For this review, use the dimensioned drawing (mm, ordinates from the lowest corner) and the shaded views. A direction names the side the tool comes from. Round coordinates to 2 decimals unless told otherwise and drop trailing zeros. Loops run counter-clockwise (first coordinate to the right, second up) from the corner with the lowest first, then second, coordinate; pieces in that order, holes last.
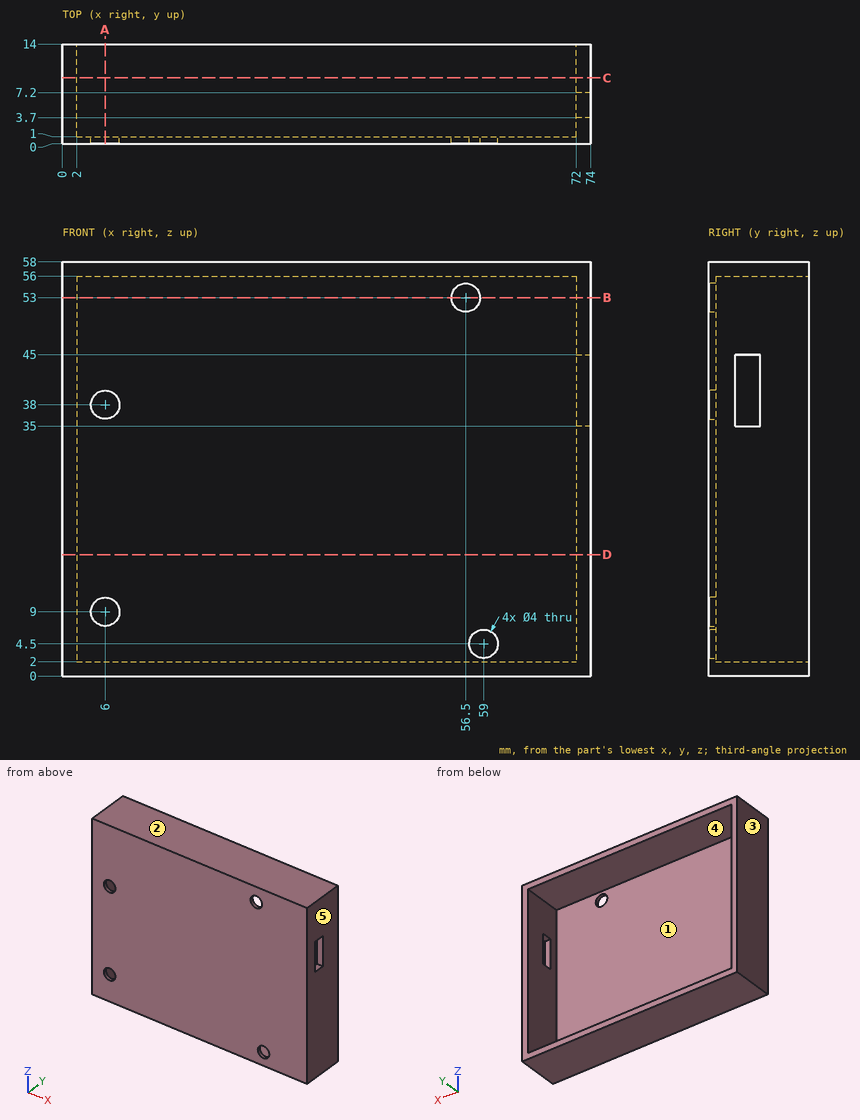
(1) Add section A-A (x = 6). Give the boundary of the cut face in (y, z).
(2) The part is to be moulded in two halves that separate along X. For the marked faces 3, 4 and 5, say which applies: pulls with the +X half, pulls with the -X half, needs draft (parallel to the pull), parting line crosses it, or undercut.
(3) For L1, parallel to X at y = 0.7, z = 9; L2, parallel to X at y = 12.75, z = 52; L3, parallel to Z at x = 56.5, y = 2, list the stretches that pass through material, from the lowest coordinate up.
(4) Add section D-D (z = 17). Give the boundary of the cut face in (x, y), plus the area to 3 significant figures.
(5) Insertion check: pin 1 Ø5 at (x, z) = (6, 9) entering from +Y; pin 2 Ø2.5 at (x, z) = (56.5, 53) entering from +Y. Each pin has a flat end and moves straight along its axis. Give the tip position at first contact, or say it passes through.
(6) For the marked faces 1 and 2, list the 3-axis set-ups (+Z, -Z, +X, -X, +Y, -Y) from which the entire face can be reached by the end or side of a thin tool; tool diameter is ignored.
(7) Add section C-C (y = 9.25). Give the boundary of the cut face in (x, z), plus the area to 3 significant figures.
(8) Add section B-B (z = 53). Give the boundary of the cut face in (x, y), plus the area to 3 significant figures.
Outcome:
1. outline: (0, 0) - (14, 0) - (14, 2) - (1, 2) - (1, 7) - (0, 7) - close; (0, 11) - (1, 11) - (1, 36) - (0, 36) - close; (0, 40) - (1, 40) - (1, 56) - (14, 56) - (14, 58) - (0, 58) - close
2. face 3: pulls with the -X half
2. face 4: undercut
2. face 5: pulls with the +X half
3. L1: x = 0 to 4, 8 to 74
3. L2: x = 0 to 2, 72 to 74
3. L3: z = 0 to 2, 56 to 58
4. outline: (0, 0) - (74, 0) - (74, 14) - (72, 14) - (72, 1) - (2, 1) - (2, 14) - (0, 14) - close
4. area: 126 mm2
5. pin 1: stops at y = 1
5. pin 2: passes through
6. face 1: +Y
6. face 2: +Z, +X, -X, +Y, -Y
7. outline: (0, 0) - (74, 0) - (74, 58) - (0, 58) - close; hole (2, 2) - (72, 2) - (72, 56) - (2, 56) - close
7. area: 512 mm2
8. outline: (0, 0) - (54.5, 0) - (54.5, 1) - (2, 1) - (2, 14) - (0, 14) - close; (58.5, 0) - (74, 0) - (74, 14) - (72, 14) - (72, 1) - (58.5, 1) - close
8. area: 122 mm2
